Could you check a few things on this model? Use its own coordinates, in mm. Give positions to 0.01 mm unless a question says otherwise; leave off trailing zeros.
(1) If I drill on probe 1 along X at (y, z) = (-1150, 3.75); probe 2 along Y at (x, z) = (335, 1.5); probe 3 along Y at (x, z) = (79.5, 1.5), over which ranges is the centre line in solid material (lowest first)?
(2) Imagine slicing it at A-A, the plane y = -1093.5. State how many separate pieces and enclosed holes the cut face has, then the cut area to 3 significant figures.
(3) Will these pins go through, and if not, where does the flat tip stop? pin 1 (3.5 mm diameter, centred on x = 65.45, y = -1169.71, fed in from -Z); pin 2 (5 mm diameter, centred on y = -874.5, z = 4, fed in from -X); pin 3 (2 mm diameter, centred on y = -993.5, z = 7, fed in from -X); pin 4 (3 mm diameter, centred on y = -1143.5, z = 5.5, fed in from -X).
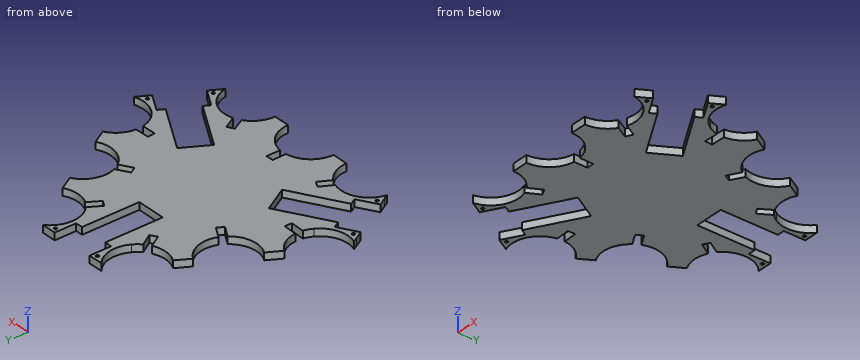
from build123d import *

# Parameters (mm, degrees)
MODEL_R            = 2
BOSS_EXTRU_1_DEPTH = 10


with BuildPart() as part:
    # Model → Boss.-Extru.1 (new body)
    with BuildSketch(Plane.XY):
        with BuildLine():
            Line((118.61641531, -1154.71765861), (127.930403211, -1137.550920057))
            Line((127.930403211, -1137.550920057), (136.72004758, -1142.319793484))
            Line((136.72004758, -1142.319793484), (127.561777994, -1159.199598646))
            add(Edge.make_bspline(
                [(127.561777994, -1159.199598646), (137.946329318, -1166.206535292), (144.775197591, -1178.081348795), (144.775197591, -1191.551327637)],
                knots=[5, 5, 5, 5, 6, 6, 6, 6], degree=3))
            Line((144.775197591, -1191.551327637), (166.775232855, -1191.551327637))
            add(Edge.make_bspline(
                [(166.775232855, -1191.551327637), (166.775232855, -1171.706328789), (181.59758393, -1155.323650906), (200.775224717, -1152.869278754)],
                knots=[7, 7, 7, 7, 8, 8, 8, 8], degree=3))
            Line((200.775224717, -1152.869278754), (200.775224717, -1133.844858588))
            Line((200.775224717, -1133.844858588), (210.775303385, -1133.844858588))
            Line((210.775303385, -1133.844858588), (210.775303385, -1152.869278754))
            add(Edge.make_bspline(
                [(210.775303385, -1152.869278754), (229.952944173, -1155.323650906), (244.775295247, -1171.706328789), (244.775295247, -1191.551327637)],
                knots=[11, 11, 11, 11, 12, 12, 12, 12], degree=3))
            Line((244.775295247, -1191.551327637), (266.775330512, -1191.551327637))
            add(Edge.make_bspline(
                [(266.775330512, -1191.551327637), (266.775330512, -1177.908060492), (273.782482476, -1165.903323825), (284.392859809, -1158.933637275)],
                knots=[13, 13, 13, 13, 14, 14, 14, 14], degree=3))
            Line((284.392859809, -1158.933637275), (275.378767469, -1142.319793484))
            Line((275.378767469, -1142.319793484), (284.168411838, -1137.550920057))
            Line((284.168411838, -1137.550920057), (293.396100097, -1154.558495198))
            add(Edge.make_bspline(
                [(293.396100097, -1154.558495198), (297.285612901, -1153.257454888), (301.447805013, -1152.551339504), (305.775189453, -1152.551339504)],
                knots=[17, 17, 17, 17, 18, 18, 18, 18], degree=3))
            add(Edge.make_bspline(
                [(305.775189453, -1152.551339504), (325.107170518, -1152.551339504), (341.150980197, -1166.618095011), (344.236752224, -1185.07381604)],
                knots=[18, 18, 18, 18, 19, 19, 19, 19], degree=3))
            Line((344.236752224, -1185.07381604), (354.349485514, -1167.558003187))
            Line((354.349485514, -1167.558003187), (328.371915256, -1152.559823052))
            Line((328.371915256, -1152.559823052), (333.130108886, -1144.318293375))
            Line((333.130108886, -1144.318293375), (264.271435112, -1104.214281331))
            Line((264.271435112, -1104.214281331), (284.368399631, -1069.09782015))
            Line((284.368399631, -1069.09782015), (353.359881836, -1109.279260715))
            Line((353.359881836, -1109.279260715), (358.371806749, -1100.598309109))
            Line((358.371806749, -1100.598309109), (384.349377007, -1115.59644618))
            Line((384.349377007, -1115.59644618), (394.422147189, -1098.149707492))
            add(Edge.make_bspline(
                [(394.422147189, -1098.149707492), (376.868524414, -1104.781903876), (356.593965223, -1097.927843343), (346.905839952, -1081.147558377)],
                knots=[28, 28, 28, 28, 29, 29, 29, 29], degree=3))
            add(Edge.make_bspline(
                [(346.905839952, -1081.147558377), (344.579194715, -1077.117744059), (343.055256727, -1072.845136637), (342.281143771, -1068.514393229)],
                knots=[29, 29, 29, 29, 30, 30, 30, 30], degree=3))
            Line((342.281143771, -1068.514393229), (322.666837131, -1069.139591932))
            Line((322.666837131, -1069.139591932), (322.348338053, -1059.144680908))
            Line((322.348338053, -1059.144680908), (341.805376085, -1058.524520657))
            add(Edge.make_bspline(
                [(341.805376085, -1058.524520657), (342.807554362, -1046.186987766), (349.649858507, -1034.529990424), (361.180765353, -1027.872601779)],
                knots=[33, 33, 33, 33, 34, 34, 34, 34], degree=3))
            Line((361.180765353, -1027.872601779), (350.180747721, -1008.820017958))
            add(Edge.make_bspline(
                [(350.180747721, -1008.820017958), (332.861563693, -1018.819235351), (311.063066514, -1014.022628906), (299.412959364, -998.355368164)],
                knots=[35, 35, 35, 35, 36, 36, 36, 36], degree=3))
            Line((299.412959364, -998.355368164), (282.706313313, -1008.121137275))
            Line((282.706313313, -1008.121137275), (277.659765191, -999.487900241))
            Line((277.659765191, -999.487900241), (294.51179427, -989.637209527))
            add(Edge.make_bspline(
                [(294.51179427, -989.637209527), (287.327047634, -971.892340888), (294.128699652, -951.115099202), (311.18088878, -941.270049832)],
                knots=[39, 39, 39, 39, 40, 40, 40, 40], degree=3))
            Line((311.18088878, -941.270049832), (300.180871148, -922.21746601))
            add(Edge.make_bspline(
                [(300.180871148, -922.21746601), (288.111668131, -929.185602268), (273.867231825, -928.967097086), (262.397130913, -922.893738254)],
                knots=[43, 43, 43, 43, 44, 44, 44, 44], degree=3))
            Line((262.397130913, -922.893738254), (252.374314615, -939.437259033))
            Line((252.374314615, -939.437259033), (243.821520562, -934.25557704))
            Line((243.821520562, -934.25557704), (254.184884548, -917.149988932))
            Line((254.184884548, -917.149988932), (254.43896034, -917.303898573))
            add(Edge.make_bspline(
                [(254.43896034, -917.303898573), (251.531472005, -914.659098768), (248.976244683, -911.528368245), (246.90591455, -907.942454481)],
                knots=[48, 48, 48, 48, 49, 49, 49, 49], degree=3))
            add(Edge.make_bspline(
                [(246.90591455, -907.942454481), (237.277044921, -891.265005615), (241.367579047, -870.433288357), (255.673338053, -858.509899007)],
                knots=[49, 49, 49, 49, 50, 50, 50, 50], degree=3))
            Line((255.673338053, -858.509899007), (247.962525336, -858.509899007))
            Line((247.962525336, -858.509899007), (235.71762245, -858.509899007))
            Line((235.71762245, -858.509899007), (235.71762245, -888.509876627))
            Line((235.71762245, -888.509876627), (225.717543782, -888.509876627))
            Line((225.717543782, -888.509876627), (225.717543782, -968.509903076))
            Line((225.717543782, -968.509903076), (185.717573622, -968.509903076))
            Line((185.717573622, -968.509903076), (185.717573622, -888.509876627))
            Line((185.717573622, -888.509876627), (175.717494954, -888.509876627))
            Line((175.717494954, -888.509876627), (175.717494954, -858.509899007))
            Line((175.717494954, -858.509899007), (163.472592068, -858.509899007))
            Line((163.472592068, -858.509899007), (155.761779351, -858.509899007))
            add(Edge.make_bspline(
                [(155.761779351, -858.509899007), (170.067538357, -870.433288357), (174.158072482, -891.265005615), (164.529202853, -907.942454481)],
                knots=[61, 61, 61, 61, 62, 62, 62, 62], degree=3))
            add(Edge.make_bspline(
                [(164.529202853, -907.942454481), (162.357759168, -911.703723605), (159.653531467, -914.965540012), (156.568103949, -917.689577013)],
                knots=[62, 62, 62, 62, 63, 63, 63, 63], degree=3))
            Line((156.568103949, -917.689577013), (156.730884711, -917.590961154))
            Line((156.730884711, -917.590961154), (167.094248697, -934.696549262))
            Line((167.094248697, -934.696549262), (158.541454644, -939.878231255))
            Line((158.541454644, -939.878231255), (148.439573405, -923.204399739))
            add(Edge.make_bspline(
                [(148.439573405, -923.204399739), (137.075236924, -928.972781494), (123.114504231, -929.064937798), (111.254246256, -922.21746601)],
                knots=[67, 67, 67, 67, 68, 68, 68, 68], degree=3))
            Line((111.254246256, -922.21746601), (100.254228624, -941.270049832))
            add(Edge.make_bspline(
                [(100.254228624, -941.270049832), (117.498998589, -951.226203532), (124.261721028, -972.363070122), (116.675965277, -990.237259033)],
                knots=[71, 71, 71, 71, 72, 72, 72, 72], degree=3))
            Line((116.675965277, -990.237259033), (133.255831814, -999.928872463))
            Line((133.255831814, -999.928872463), (128.209283691, -1008.562109497))
            Line((128.209283691, -1008.562109497), (111.632173231, -998.872089423))
            add(Edge.make_bspline(
                [(111.632173231, -998.872089423), (99.89077105, -1014.127489), (78.381834147, -1018.708604723), (61.254197428, -1008.819974894)],
                knots=[75, 75, 75, 75, 76, 76, 76, 76], degree=3))
            Line((61.254197428, -1008.819974894), (50.254179796, -1027.872558716))
            add(Edge.make_bspline(
                [(50.254179796, -1027.872558716), (61.92823036, -1034.612500461), (68.798784288, -1046.476375786), (69.666603841, -1058.983192057)],
                knots=[79, 79, 79, 79, 80, 80, 80, 80], degree=3))
            Line((69.666603841, -1058.983192057), (88.567431206, -1059.58565313))
            Line((88.567431206, -1059.58565313), (88.248759874, -1069.580564155))
            Line((88.248759874, -1069.580564155), (69.068879774, -1068.969231961))
            add(Edge.make_bspline(
                [(69.068879774, -1068.969231961), (68.270995659, -1073.144084798), (66.77444618, -1077.258906847), (64.529277452, -1081.147558377)],
                knots=[83, 83, 83, 83, 84, 84, 84, 84], degree=3))
            add(Edge.make_bspline(
                [(64.529277452, -1081.147558377), (54.876636664, -1097.866434516), (34.714904351, -1104.731734673), (17.205723307, -1098.222140625)],
                knots=[84, 84, 84, 84, 85, 85, 85, 85], degree=3))
            Line((17.205723307, -1098.222140625), (21.089379448, -1104.948818752))
            Line((21.089379448, -1104.948818752), (27.24318126, -1115.607384359))
            Line((27.24318126, -1115.607384359), (53.239699544, -1100.598309109))
            Line((53.239699544, -1100.598309109), (58.239566623, -1109.258590142))
            Line((58.239566623, -1109.258590142), (127.521642632, -1069.258576918))
            Line((127.521642632, -1069.258576918), (147.521627712, -1103.899571859))
            Line((147.521627712, -1103.899571859), (78.239551703, -1143.899628146))
            Line((78.239551703, -1143.899628146), (83.239591037, -1152.559823052))
            Line((83.239591037, -1152.559823052), (57.243245008, -1167.568898302))
            Line((57.243245008, -1167.568898302), (63.432359049, -1178.288829671))
            Line((63.432359049, -1178.288829671), (67.321699598, -1185.02567083))
            add(Edge.make_bspline(
                [(67.321699598, -1185.02567083), (70.427280924, -1166.593634833), (86.460066297, -1152.551339504), (105.775166395, -1152.551339504)],
                knots=[0, 0, 0, 0, 1, 1, 1, 1], degree=3))
            add(Edge.make_bspline(
                [(105.775166395, -1152.551339504), (110.274633355, -1152.551339504), (114.594955349, -1153.315763129), (118.61641531, -1154.71765861)],
                knots=[1, 1, 1, 1, 2, 2, 2, 2], degree=3))
        make_face()
        with Locations((65.451386675, -1169.708192825)):
            Circle(MODEL_R, mode=Mode.SUBTRACT)
        with Locations((29.494548276, -1107.429239443)):
            Circle(MODEL_R, mode=Mode.SUBTRACT)
        with Locations((169.760752604, -864.530547878)):
            Circle(MODEL_R, mode=Mode.SUBTRACT)
        with Locations((241.6743648, -864.530504815)):
            Circle(MODEL_R, mode=Mode.SUBTRACT)
        with Locations((382.116933599, -1107.429281733)):
            Circle(MODEL_R, mode=Mode.SUBTRACT)
        with Locations((346.16022151, -1169.708251653)):
            Circle(MODEL_R, mode=Mode.SUBTRACT)
    extrude(amount=BOSS_EXTRU_1_DEPTH)


solid = part.part
Answer block:
1. probe 1: x = 81.76 to 121.18, 132.55 to 200.78, 210.78 to 279.55, 290.92 to 329.85
1. probe 2: y = -1165.73 to -1156.39, -1098.59 to -1068.75, -1058.74 to -1013.81
1. probe 3: y = -1162.73 to -1154.72, -1146.08 to -1143.17, -1096.98 to -1069.3, -1059.3 to -1014.03
2. separate pieces: 3
2. enclosed holes: 0
2. area: 1,930 mm2
3. pin 1: passes through
3. pin 2: stops at x = 166.12
3. pin 3: stops at x = 120.55
3. pin 4: stops at x = 78.24
